Geometry check sheet. Reference: the model listing, model coordinates, mm. A direction names the side the tool comes from. Coordinates: 2 decimals unless noted, no trailing zeros. Order: outer loops, then holes, each group sorted by start corner. A loop starts at its lowest first (then second) coordinate and runs counter-clockwise, first axis right, second up. Notation, with made-up numbers: (11, 86.25) - (29, 86.25) arc R8 cw to (29, 101.25) - close; hole circle Ø6 at (89, 8.5). An arc over 180 degrees is marked (long way). Return JSON: item names as keys, results as strings. Group by question number.
Item 1: Section check C-C on x = -19. Enter the section's corners in (y, z).
Item 2: Draft check along Z on faces 1 (the cylindrical face through (20.12, 26.72, -1.08)), 2 (the flat face through (25, 7, 0)), 3 (the flat face through (0, 7, 0)). Enter one of: pulls with the +Z half, pulls with the -Z half, needs draft (parallel to the pull), parting line crosses it, or undercut.
Item 3: Section check B-B on y = 11.5. Enter the section's corners in (x, z).
Item 4: Section check A-A on z = 0. Enter the section's corners in (x, y).
Item 5: Gauge pin test, flat ends, axial feed: pin 1 (4 mm diameter, centred on x = 25, z = 0.5, fed in from -Y); pin 2 (8 mm diameter, centred on x = 0.5, z = -5, fed in from +Y); pin 3 (10 mm diameter, centred on y = 39.5, z = -2.5, fed in from -X). Record the tip position at first contact, or that the pin passes through.
Item 6: Scan lines: probe 1 along X at (y, z) = (2.5, 0); probe 2 along Y at (x, z) = (-22.5, -6); probe 3 along X at (y, z) = (2, -2.25). Record each from-to range of solid material in increasing order.
Item 7: Section check D-D on z = 6.5. Enter the section's corners in (x, y), then the cut area to 3 significant figures.
Item 8: Tool access check on faces 4 (the cylindrical face through (-34, 3, 0)), 5 (the cylindrical face through (28.966, 3.451, -0.521)). Record the directions out of +Z, -Z, +X, -X, +Y, -Y that give a thin tool (end or side, any length) a straight path to the whole face; none if there is none.
from build123d import *

# Parameters (mm, degrees)
SKETCH1_R           = 4
SKETCH1_R_2         = 3
BOSS_EXTRUDE1_DEPTH = 7
SKETCH2_R           = 5
BOSS_EXTRUDE2_DEPTH = 40


with BuildPart() as part:
    # Sketch1 → Boss-Extrude1 (new body)
    with BuildSketch(Plane(origin=(0, 0, 0), x_dir=(1, 0, 0), z_dir=(0, 1, 0))):
        with BuildLine():
            Line((-25, 9), (25, 9))
            ThreePointArc((25, 9), (34, 0), (25, -9))
            Line((25, -9), (-25, -9))
            ThreePointArc((-25, -9), (-34, 0), (-25, 9))
        make_face()
        with Locations(Location((25, 0, 0), (0, 0, 270))):  # turned: the seam where the file's is
            Circle(SKETCH1_R, mode=Mode.SUBTRACT)
        with Locations(Location((-25, 0, 0), (0, 0, 270))):  # turned: the seam where the file's is
            Circle(SKETCH1_R_2, mode=Mode.SUBTRACT)
    extrude(amount=BOSS_EXTRUDE1_DEPTH)

    # Sketch2 → Boss-Extrude2 (add)
    with BuildSketch(Plane(origin=(0, 7, 0), x_dir=(1, 0, 0), z_dir=(0, 1, 0))):
        with Locations(Location((25, 0, 0), (0, 0, 270))):  # turned: the seam where the file's is
            Circle(SKETCH2_R)
    extrude(amount=BOSS_EXTRUDE2_DEPTH)


solid = part.part
Computed:
{
 "1": {"outline": "(0, -9) - (7, -9) - (7, 9) - (0, 9) - close"},
 "2": {"face 1": "parting line crosses it", "face 2": "undercut", "face 3": "needs draft"},
 "3": {"outline": "circle Ø10 at (25, 0)"},
 "4": {"outline": "(-34, 0) - (-28, 0) - (-28, 7) - (-34, 7) - close; (-22, 0) - (21, 0) - (21, 7) - (29, 7) - (29, 0) - (34, 0) - (34, 7) - (30, 7) - (30, 47) - (20, 47) - (20, 7) - (-22, 7) - close"},
 "5": {"pin 1": "stops at y = 7", "pin 2": "stops at y = 7", "pin 3": "stops at x = 20"},
 "6": {"probe 1": "x = -34 to -28, -22 to 21, 29 to 34", "probe 2": "y = 0 to 7", "probe 3": "x = -33.71 to -26.98, -23.02 to 21.69, 28.31 to 33.71"},
 "7": {"outline": "(-31.22, 0) - (31.22, 0) - (31.22, 7) - (-31.22, 7) - close", "area": "437 mm²"},
 "8": {"face 4": "-X, +Y, -Y", "face 5": "-Y"}
}
